Read the model definition and answer for the solid it produces. Units are mm, in the model's axes. Face numbers are marked on the shaded views. A direction names the side the tool comes from. Round coordinates to 2 decimals unless told otherwise and drop trailing zeros. Order: outer loops, then holes, each group sorted by start corner. A loop starts at its lowest first (then second) coordinate and runs counter-clockwise, first axis right, second up. Notation, with made-up numbers: (77.5, 62.25) -> (113.5, 62.25) arc R38 cw to (113.5, 100.25) -> close; hole circle Ø7 at (-36.5, 9.5). An arc over 180 degrees is marked (long way). Answer as a JSON object with one key per item and string values. Group by question number.
Item 1: For the marked faces 1, 2 and 3, determine the directions among +Z, -Z, +X, -X, +Y, -Y from which every point of the face is accessible in a straight line to the end or side of a thin tool.
Item 2: The mould has two halves that part along Z. Classify the marked faces 4, 5 and 6: pulls with the +Z half, pulls with the -Z half, needs draft (parallel to the pull), parting line crosses it, or undercut.
Item 3: Consider probe 1 along Y at (x, z) = (-6.25, 3.25); probe 2 along X at (y, z) = (6.5, 0); probe 3 along Y at (x, z) = (7, -6). Determine where each line is inside the solid, lowest interval first. Write a range as from..to.
Item 4: Given P1, Ø6, axis at x = 7, y = 3, coming from the -Z side; P2, Ø8, axis at x = 1, z = 2, coming from the +Y side; P3, Ø8, axis at x = 7, z = -5, coming from the -Y side; P4, Ø2, axis at y = 15, z = 4, coming from the -X side, each flat-ended and moving along its own axis, determine where each tip first touches the part or whether it passes through.
Item 5: Section C-C, the plane x = 7.5 is taken. Write down the section's boundary in (y, z), plus the area to 3 significant figures.
Item 6: Section D-D, the plane z = -6.5 is taken. Write down the section's boundary in (x, y).
Item 7: Section B-B, the plane y = 9.25 is taken. Write down the section's boundary in (x, z).
from build123d import *

# Parameters (mm, degrees)
CHANFREIN1_SIZE         = 0.5
ESQUISSE2_R             = 12.5
ENL_V_MAT_EXTRU_1_DEPTH = 21.820662814
ESQUISSE3_R             = 8.05
ESQUISSE3_R_2           = 6.05
ENL_V_MAT_EXTRU_2_DEPTH = 1.2


with BuildPart() as part:
    # Esquisse1 → Révolution1 (revolve)
    with BuildSketch(Plane.XY, mode=Mode.PRIVATE) as r_volution1_sk:
        Polygon((0.65, 0), (0.65, 2.5), (1.75, 3.6), (1.75, 16.75), (3, 18), (4.475, 18), (4.475, 15.5), (5, 15.5), (5, 11), (12.5, 11), (12.5, 7), (3.914153607, 7), align=None)
    revolve(r_volution1_sk.sketch.rotate(Axis((0, 0, 0), (0, 1, 0)), 90), axis=Axis((0, 0, 0), (0, 1, 0)))

    # Chanfrein1
    chanfrein1_edges = [part.edges().sort_by_distance(p)[0] for p in [
        (0, 15.5, 5),
    ]]
    chamfer(chanfrein1_edges, length=CHANFREIN1_SIZE)

    # Esquisse2 → Enlèv. mat.-Extru.1 (cut, through all)
    with BuildSketch(Plane(origin=(0, 11, 0), x_dir=(1, 0, 0), z_dir=(0, 1, 0))):
        Circle(ESQUISSE2_R)
        Polygon((-10.911920088, 0), (-5.455960044, 9.45), (5.455960044, 9.45), (10.911920088, 0), (5.455960044, -9.45), (-5.455960044, -9.45), align=None, mode=Mode.SUBTRACT)
    extrude(amount=-ENL_V_MAT_EXTRU_1_DEPTH, mode=Mode.SUBTRACT)

    # Esquisse3 → Enlèv. mat.-Extru.2 (cut)
    with BuildSketch(Plane(origin=(0, 11, 0), x_dir=(1, 0, 0), z_dir=(0, 1, 0))):
        with Locations(Location((0, 0, 0), (0, 0, 270))):
            Circle(ESQUISSE3_R)
        with Locations(Location((0, 0, 0), (0, 0, 270))):
            Circle(ESQUISSE3_R_2, mode=Mode.SUBTRACT)
    extrude(amount=-ENL_V_MAT_EXTRU_2_DEPTH, mode=Mode.SUBTRACT)


solid = part.part
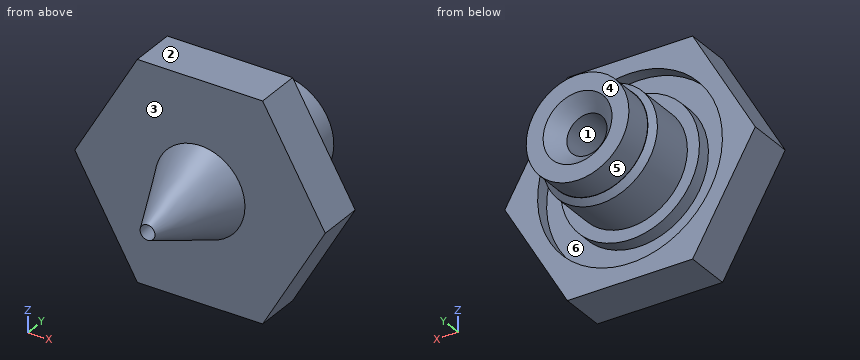
Values found:
{
 "1": {"face 1": "+Y", "face 2": "+Z, +X, -X, +Y, -Y", "face 3": "-Y"},
 "2": {"face 4": "needs draft", "face 5": "parting line crosses it", "face 6": "undercut"},
 "3": {"probe 1": "7..9.8", "probe 2": "-3.68..-1.75, 1.75..3.68", "probe 3": "7..11"},
 "4": {"P1": "through", "P2": "y = 18", "P3": "y = 7", "P4": "x = -4"},
 "5": {"outline": "(7, -5.91) -> (11, -5.91) -> (11, -2.92) -> (9.8, -2.92) -> (9.8, 2.92) -> (11, 2.92) -> (11, 5.91) -> (7, 5.91) -> close", "area": "40.3 mm2"},
 "6": {"outline": "(-7.16, 7) -> (7.16, 7) -> (7.16, 11) -> (4.75, 11) -> (4.75, 9.8) -> (-4.75, 9.8) -> (-4.75, 11) -> (-7.16, 11) -> close"},
 "7": {"outline": "(-10.91, 0) -> (-5.46, -9.45) -> (5.46, -9.45) -> (10.91, 0) -> (5.46, 9.45) -> (-5.46, 9.45) -> close; hole circle Ø3.5 at (0, 0)"}
}
